Drawing for the job (mm, zero at the part's lowest x, y, z). A direction names the side the tool comes from. Coordinates: 2 decimals unless noted, no trailing zeros. Write each loop counter-clockwise with the first axis right and the second up, starting at its lowest first coordinate (ties: lowest second). Pieces come first, ordered by that corner, then holes. Notation, with made-up numbers: (50.5, 81.5) -> (97.5, 81.5) arc R26 cw to (97.5, 111.5) -> close; hole circle Ø2 at (88.5, 19). An arc over 180 degrees is marked (long way). Answer as CSV lines item,"result".
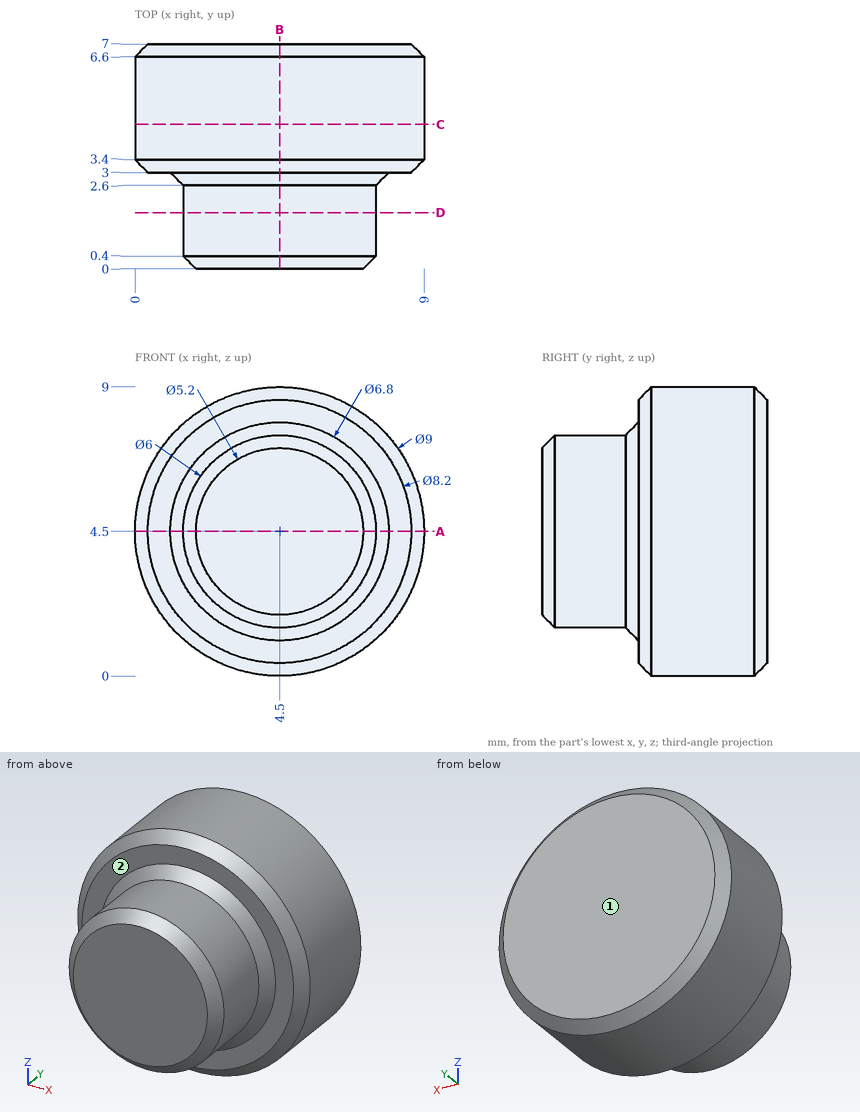
Item 1: Flat gauge pins, fed straight in: pin 1 (1.5 mm diameter, centred on y = 2, z = 6, fed in from +X); pin 2 (2 mm diameter, centred on y = 5, z = 6.5, fed in from -X); pin 3 (1.5 mm diameter, centred on x = 3.5, y = 4, fed in from +Z). Where does each tip first touch, or does it go through?
Answer below:
pin 1,"stops at x = 7.4"
pin 2,"stops at x = 0.11"
pin 3,"stops at z = 8.99"
Item 2: Saw through at B-B on x = 4.5. Give the cut face in (y, z), and give its area (3 significant figures).
Answer below:
outline,"(0, 1.9) -> (0.4, 1.5) -> (2.6, 1.5) -> (3, 1.1) -> (3, 0.4) -> (3.4, 0) -> (6.6, 0) -> (7, 0.4) -> (7, 8.6) -> (6.6, 9) -> (3.4, 9) -> (3, 8.6) -> (3, 7.9) -> (2.6, 7.5) -> (0.4, 7.5) -> (0, 7.1) -> close"
area,"53.7 mm2"
Item 3: 3-axis set-ups, long thin cutter, end or side, ignore diameter. For the marked faces 1 and 2: which of +Z, -Z, +X, -X, +Y, -Y reach the whole face in a straight line?
Answer below:
face 1,"+Z, -Z, +X, -X, +Y"
face 2,"-Y"
Item 4: Saw through at A-A on z = 4.5. Give the cut face in (x, y).
Answer below:
outline,"(0, 3.4) -> (0.4, 3) -> (1.1, 3) -> (1.5, 2.6) -> (1.5, 0.4) -> (1.9, 0) -> (7.1, 0) -> (7.5, 0.4) -> (7.5, 2.6) -> (7.9, 3) -> (8.6, 3) -> (9, 3.4) -> (9, 6.6) -> (8.6, 7) -> (0.4, 7) -> (0, 6.6) -> close"
Item 5: Saw through at C-C on y = 4.5. Give the cut face in (x, z), and give its area (3 significant figures).
Answer below:
outline,"circle Ø9 at (4.5, 4.5)"
area,"63.6 mm2"
Item 6: Wall check: line 1 (Y direction, x = 7.25, z = 1.5); line 2 (X direction, y = 4.5, z = 4); line 3 (Z direction, x = 7.5, y = 4.25). Give the ranges that are in metal, low to high. Write a range as from..to.
Answer below:
line 1,"y = 3..7"
line 2,"x = 0.03..8.97"
line 3,"z = 1.15..7.85"
Item 7: Saw through at D-D on y = 1.75. Give the cut face in (x, z).
Answer below:
outline,"circle Ø6 at (4.5, 4.5)"
